The drawing under review shows one solid part. Ordinate dimensions are in mm from its lowest x, y, z. Give positions to 0.01 mm unless a question says otherwise; leave off trailing zeros. Order: outer loops, then holes, each group sorted by start corner. A loop starts at its lowest first (then second) coordinate and runs counter-clockwise, first axis right, second up. Notation, with made-up numbers: (14.25, 73) - (59.25, 73) arc R18 ccw to (59.25, 91) - close; hole circle Ø4 at (-37, -11.5). An arc over 180 degrees is marked (long way). Write item = value, one per line. Start each with the question number.
1. We need section A-A, the plane x = 3.5. Give the boundary of the cut face in (y, z).
2. We need section C-C, the plane z = 1.5. Give the boundary of the cut face in (x, y).
3. For P1, Ø1.5, axis at x = 1.5, z = 6, coming from the +Y side, flat-tipped, find the tip position at first contact; note if it passes through.
4. We need section B-B, the plane y = 84.5. Give the boundary of the cut face in (x, z).
5. Wall thickness on probe 1 along Z at (x, y) = (4.25, 103); probe 2 along Z at (x, y) = (5, 48); probe 3 along Y at (x, z) = (6, 7.25) (1 decimal): over which ranges is each line inside the solid? List them lowest first.
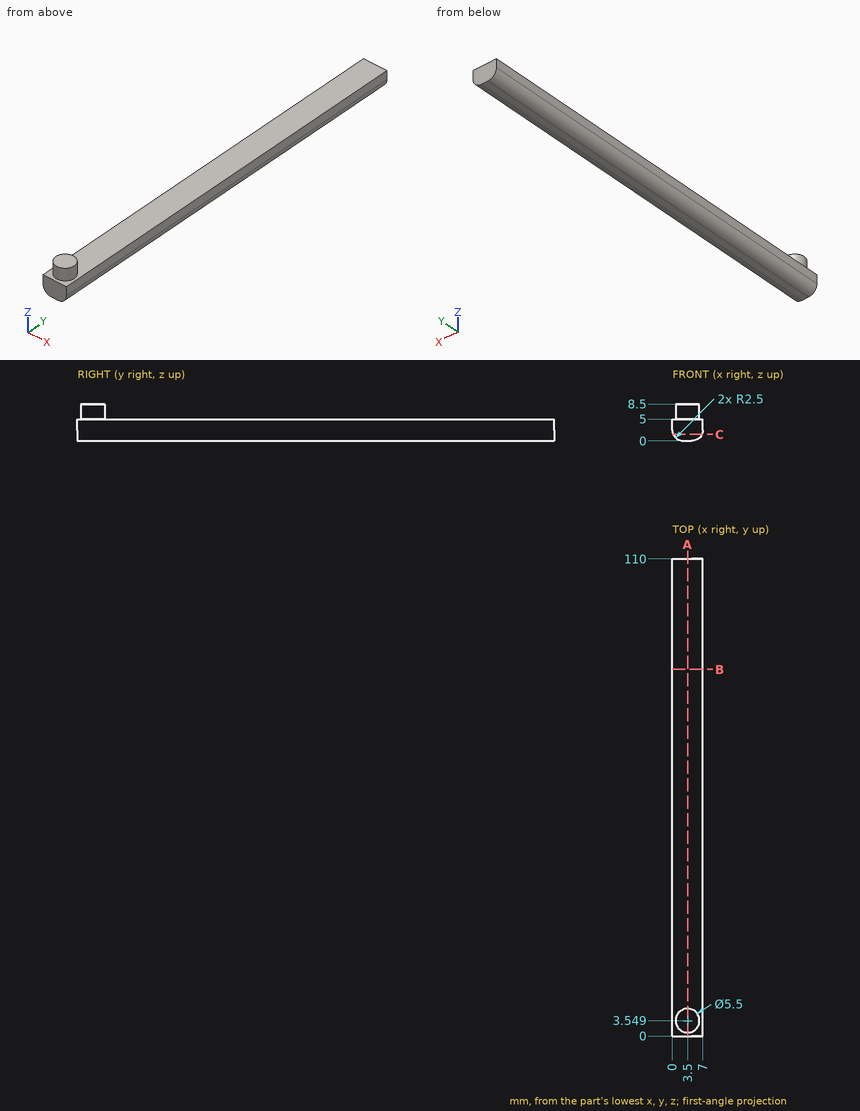
Model answer:
q1.outline = (0, 0) - (110, 0) - (110, 5) - (6.3, 5) - (6.3, 8.5) - (0.8, 8.5) - (0.8, 5) - (0, 5) - close
q2.outline = (0.21, 0) - (6.79, 0) - (6.79, 110) - (0.21, 110) - close
q3.P1 = 6
q4.outline = (0, 2.5) arc R2.5 ccw to (2.5, 0) - (4.5, 0) arc R2.5 ccw to (7, 2.5) - (7, 5) - (0, 5) - close
q5.probe_1 = 0 to 5
q5.probe_2 = 0.05 to 5
q5.probe_3 = 2.4 to 4.7
